The listing builds one solid part. Answer for the finished solid, in the listing's coordinates (mm). A direction names the side the tool comes from. Give positions to 0.01 mm unless a question says otherwise; leave off trailing zeros. Loops run counter-clockwise (first coordinate to the right, second up) from the corner with the lowest first, then second, coordinate; pieces in that order, holes last.
Item 1: Section B-B, the plane x = 64.56 is taken. Give the vertices of the cut face in (y, z), and give its area (3 significant figures).
Item 2: The mould has two halves that part along X. Classify faces 1 (the face through (37, 0, 6)), 2 (the face through (74.4, -44.43, 6.44)), 3 (the face through (0.57, -0.6, 6.44)), 4 (the face through (37, -2, 6)): pulls with the +X half, pulls with the -X half, needs draft (parallel to the pull), parting line crosses it, or undercut.
Item 3: Section C-C, the plane z = 11.5 is taken. Give the vertices of the cut face in (x, y) (3 decimals).
Item 4: Section A-A, the plane y = -8.35 is taken. Give the vertices of the cut face in (x, z) (3 decimals), and give its area (3 significant figures).
Item 5: Each of these flat-tipped pins is pushed along its axis until it touches: pin 1 Ø4 at (x, y) = (10.44, -8.35) entering from +Z; pin 2 Ø10 at (x, y) = (9.5, -37) entering from -Z; pin 3 Ø4 at (x, y) = (66.5, -8.5) entering from -Z; pin 4 Ø8.5 at (x, y) = (64.56, -8.35) entering from -Z. Where does it stop, or does it pass through?
Item 6: A tool of negligible diameter and unlimited length cuts with its end or side. For faces 5 (the face through (38, -14.7, 6)), 6 (the face through (66.137, -11.382, 3.475)), from which of +Z, -Z, +X, -X, +Y, -Y can it reach the whole face along a straight path? Write none if from no direction.
Item 7: Consider line 1 along X through (y, z) = (-8.35, 6.5) (3 decimals); line 2 along X through (y, z) = (-12, 7.75) (3 decimals); line 3 along Y through (x, z) = (10.44, 5.75). Determine where each line is inside the solid, lowest interval first.
Item 8: Section D-D, the plane x = 32.5 is taken. Give the vertices of the cut face in (y, z), and give its area (3 significant figures).
from build123d import *

# Parameters (mm, degrees)
SKETCH1_W                                        = 75
SKETCH1_H                                        = 45
BOSS_EXTRUDE1_DEPTH                              = 12.7
CSK_FOR_1_4_FLAT_HEAD_MACHINE_SCREW2_D           = 6.5278
CSK_FOR_1_4_FLAT_HEAD_MACHINE_SCREW2_CSINK_D     = 12.8778
CSK_FOR_1_4_FLAT_HEAD_MACHINE_SCREW2_CSINK_ANGLE = 82
FILLET1_R                                        = 2
FILLET2_R                                        = 2


with BuildPart() as part:
    # Sketch1 → Boss-Extrude1 (new body)
    with BuildSketch(Plane.XY):
        with Locations((37.5, -22.5)):
            Rectangle(SKETCH1_W, SKETCH1_H)
        Polygon((37.5, -2), (53.375, -2), (53.375, -14.7), (21.625, -14.7), (21.625, -2), align=None, mode=Mode.SUBTRACT)
    extrude(amount=BOSS_EXTRUDE1_DEPTH)

    # CSK for 1/4 Flat Head Machine Screw2 (through all)
    with Locations(Plane(origin=(0, 0, 0), x_dir=(-1, 0, 0), z_dir=(0, 0, -1))):
        with Locations((-64.56, -8.35), (-10.44, -8.35)):
            CounterSinkHole(CSK_FOR_1_4_FLAT_HEAD_MACHINE_SCREW2_D / 2, CSK_FOR_1_4_FLAT_HEAD_MACHINE_SCREW2_CSINK_D / 2, counter_sink_angle=CSK_FOR_1_4_FLAT_HEAD_MACHINE_SCREW2_CSINK_ANGLE)

    # Fillet1
    fillet1_edges = [part.edges().sort_by_distance(p)[0] for p in [
        (0, 0, 6.35),
        (0, -45, 6.35),
    ]]
    fillet(fillet1_edges, radius=FILLET1_R)

    # Fillet2
    fillet2_edges = [part.edges().sort_by_distance(p)[0] for p in [
        (75, 0, 6.35),
        (75, -45, 6.35),
    ]]
    fillet(fillet2_edges, radius=FILLET2_R)


solid = part.part
Worked answers:
1. outline: (-45, 0) - (-14.79, 0) - (-11.61, 3.65) - (-11.61, 12.7) - (-45, 12.7) - close; (-5.09, 3.65) - (-1.91, 0) - (0, 0) - (0, 12.7) - (-5.09, 12.7) - close
1. area: 477 mm2
2. face 1: needs draft
2. face 2: pulls with the +X half
2. face 3: pulls with the -X half
2. face 4: undercut
3. outline: (0, -43) arc R2 ccw to (2, -45) - (73, -45) arc R2 ccw to (75, -43) - (75, -2) arc R2 ccw to (73, 0) - (2, 0) arc R2 ccw to (0, -2) - close; hole circle Ø6.528 at (10.44, -8.35); hole (21.625, -14.7) - (53.375, -14.7) - (53.375, -2) - (21.625, -2) - close; hole circle Ø6.528 at (64.56, -8.35)
4. outline: (0, 0) - (4.001, 0) - (7.176, 3.652) - (7.176, 12.7) - (0, 12.7) - close; (13.704, 3.652) - (16.879, 0) - (21.625, 0) - (21.625, 12.7) - (13.704, 12.7) - close; (53.375, 0) - (58.121, 0) - (61.296, 3.652) - (61.296, 12.7) - (53.375, 12.7) - close; (67.824, 3.652) - (70.999, 0) - (75, 0) - (75, 12.7) - (67.824, 12.7) - close
4. area: 360 mm2
5. pin 1: passes through
5. pin 2: stops at z = 0
5. pin 3: stops at z = 2.87
5. pin 4: stops at z = 2.52
6. face 5: +Z, -Z
6. face 6: -Z
7. line 1: x = 0 to 7.176, 13.704 to 21.625, 53.375 to 61.296, 67.824 to 75
7. line 2: x = 0 to 21.625, 53.375 to 75
7. line 3: y = -45 to -11.61, -5.09 to 0
8. outline: (-45, 0) - (-14.7, 0) - (-14.7, 12.7) - (-45, 12.7) - close; (-2, 0) - (0, 0) - (0, 12.7) - (-2, 12.7) - close
8. area: 410 mm2
